Geometry: final body of the model. Coordinates: model frame, mm. A direction names the side the tool comes from. Coordinates: 2 decimals unless noted, no trailing zeros. Write each loop counter-clockwise with the first axis right and the second up, starting at its lowest first coordinate (ties: lowest second). Pieces come first, ordered by that corner, then holes. Notation, with made-up numbers: (4, -1) - (13, -1) arc R16 cw to (13, 8) - close; hole circle Ø4 at (4, 21). An arc over 180 degrees is marked (long way). Put each result on its own line as item: value.
```python
from build123d import *

# Parameters (mm, degrees)
Y_PCB_EXTR_DEPTH                = 1.6
SKETCH1_5_R                     = 1.524
Z0X0_CORNER_EXTR_DEPTH          = 1.6
SKETCH1_6_R                     = 1.524
Z0X_CORNER_EXTR_DEPTH           = 1.6
SKETCH1_7_R                     = 1.524
Z_X0_CORNER_EXTR_DEPTH          = 1.6
SKETCH1_8_R                     = 1.524
Z_X_CORNER_EXTR_DEPTH           = 1.6
Y_DISPLAY_EXTR_DEPTH            = 5.6
SKETCH1_11_W                    = 11.43
SKETCH1_11_H                    = 13.952
Y_DISPLAY_EXTR_BEHIND_USD_DEPTH = 5.6
SKETCH1_12_W                    = 11.43
SKETCH1_12_H                    = 3.048
Y_USD_EXTR_OUTER_EDGE_DEPTH     = 1.6
SKETCH1_13_W                    = 11.43
SKETCH1_13_H                    = 13.952
Y_USD_EXTR_DEPTH                = 2
SKETCH1_14_W                    = 11.43
SKETCH1_14_H                    = 3.048
Y_USD_EXTR_OUTER_BOTTOM_DEPTH   = 2


with BuildPart() as part:
    # Sketch1 → Y_ PCB extr (new body)
    with BuildSketch(Plane(origin=(0, 0, 0), x_dir=(1, 0, 0), z_dir=(0, 1, 0))):
        Polygon((81.28, 50.8), (76.2, 50.8), (66.167, 50.8), (66.167, 47.752), (73.152, 47.752), (73.152, 3.048), (13.716, 3.048), (13.716, 47.752), (54.737, 47.752), (54.737, 50.8), (5.08, 50.8), (0, 50.8), (0, 0), (5.08, 0), (76.2, 0), (81.28, 0), align=None)
    extrude(amount=Y_PCB_EXTR_DEPTH)

    # Sketch1_5 → Z0X0 corner extr (add)
    with BuildSketch(Plane(origin=(0, 0, 0), x_dir=(1, 0, 0), z_dir=(0, 1, 0))):
        with BuildLine():
            Line((0, 50.8), (5.08, 50.8))
            Line((5.08, 50.8), (5.08, 53.98))
            ThreePointArc((5.08, 53.98), (2.54, 56.52), (0, 53.98))
            Line((0, 53.98), (0, 50.8))
        make_face()
        with Locations(Location((2.54, 53.98, 0), (0, 0, 270))):
            Circle(SKETCH1_5_R, mode=Mode.SUBTRACT)
    extrude(amount=Z0X0_CORNER_EXTR_DEPTH)

    # Sketch1_6 → Z0X_ corner extr (add)
    with BuildSketch(Plane(origin=(0, 0, 0), x_dir=(1, 0, 0), z_dir=(0, 1, 0))):
        with BuildLine():
            Line((76.2, 53.98), (76.2, 50.8))
            Line((76.2, 50.8), (81.28, 50.8))
            Line((81.28, 50.8), (81.28, 53.98))
            ThreePointArc((81.28, 53.98), (78.74, 56.52), (76.2, 53.98))
        make_face()
        with Locations(Location((78.74, 53.98, 0), (0, 0, 270))):
            Circle(SKETCH1_6_R, mode=Mode.SUBTRACT)
    extrude(amount=Z0X_CORNER_EXTR_DEPTH)

    # Sketch1_7 → Z_X0 corner extr (add)
    with BuildSketch(Plane(origin=(0, 0, 0), x_dir=(1, 0, 0), z_dir=(0, 1, 0))):
        with BuildLine():
            Line((5.08, -3.18), (5.08, 0))
            Line((5.08, 0), (0, 0))
            Line((0, 0), (0, -3.18))
            ThreePointArc((0, -3.18), (2.54, -5.72), (5.08, -3.18))
        make_face()
        with Locations(Location((2.54, -3.18, 0), (0, 0, 270))):
            Circle(SKETCH1_7_R, mode=Mode.SUBTRACT)
    extrude(amount=Z_X0_CORNER_EXTR_DEPTH)

    # Sketch1_8 → Z_X_ corner extr (add)
    with BuildSketch(Plane(origin=(0, 0, 0), x_dir=(1, 0, 0), z_dir=(0, 1, 0))):
        with BuildLine():
            Line((81.28, -3.18), (81.28, 0))
            Line((81.28, 0), (76.2, 0))
            Line((76.2, 0), (76.2, -3.18))
            ThreePointArc((76.2, -3.18), (78.74, -5.72), (81.28, -3.18))
        make_face()
        with Locations(Location((78.74, -3.18, 0), (0, 0, 270))):
            Circle(SKETCH1_8_R, mode=Mode.SUBTRACT)
    extrude(amount=Z_X_CORNER_EXTR_DEPTH)

    # Sketch1_10 → Y_ display extr (add)
    with BuildSketch(Plane(origin=(0, 0, 0), x_dir=(1, 0, 0), z_dir=(0, 1, 0))):
        Polygon((73.152, 47.752), (66.167, 47.752), (66.167, 33.8), (54.737, 33.8), (54.737, 47.752), (13.716, 47.752), (13.716, 3.048), (73.152, 3.048), align=None)
    extrude(amount=Y_DISPLAY_EXTR_DEPTH)

    # Sketch1_11 → Y_ display extr behind uSD (add)
    with BuildSketch(Plane(origin=(0, 0, 0), x_dir=(1, 0, 0), z_dir=(0, 1, 0))):
        with Locations((60.452, 40.776)):
            Rectangle(SKETCH1_11_W, SKETCH1_11_H)
    extrude(amount=Y_DISPLAY_EXTR_BEHIND_USD_DEPTH)

    # Sketch1_12 → Y- uSD extr outer edge (add)
    with BuildSketch(Plane(origin=(0, 0, 0), x_dir=(1, 0, 0), z_dir=(0, 1, 0))):
        with Locations((60.452, 49.276)):
            Rectangle(SKETCH1_12_W, SKETCH1_12_H)
    extrude(amount=Y_USD_EXTR_OUTER_EDGE_DEPTH)

    # Sketch1_13 → Y- uSD extr (add)
    with BuildSketch(Plane(origin=(0, 0, 0), x_dir=(1, 0, 0), z_dir=(0, 1, 0))):
        with Locations((60.452, 40.776)):
            Rectangle(SKETCH1_13_W, SKETCH1_13_H)
    extrude(amount=-Y_USD_EXTR_DEPTH)

    # Sketch1_14 → Y- uSD extr outer bottom (add)
    with BuildSketch(Plane(origin=(0, 0, 0), x_dir=(1, 0, 0), z_dir=(0, 1, 0))):
        with Locations((60.452, 49.276)):
            Rectangle(SKETCH1_14_W, SKETCH1_14_H)
    extrude(amount=-Y_USD_EXTR_OUTER_BOTTOM_DEPTH)


solid = part.part
```
1. Mould query, pull axis X, two halves, no side actions, for faces 1 (the flat face through (48, 1, -50.8)), 2 (the flat face through (0, 1, -26)), 3 (the flat face through (43, 4, -47.752)), 4 (the flat face through (73.152, 4, -25)). Classes: +X half, -X half, draft (parallel to the pull), parting line (faces both ways), or undercut.
Answer below:
face 1: undercut
face 2: -X half
face 3: draft
face 4: +X half
2. Section query B-B (z = -14). Return loops of the section in (x, y), then the cut area to 3 significant figures.
Answer below:
outline: (0, 0) - (81.28, 0) - (81.28, 1.6) - (73.15, 1.6) - (73.15, 5.6) - (13.72, 5.6) - (13.72, 1.6) - (0, 1.6) - close
area: 368 mm²
3. Section query A-A (x = 78.74). Return loops of the section in (y, z).
Answer below:
outline: (0, -56.52) - (1.6, -56.52) - (1.6, -55.5) - (0, -55.5) - close; (0, -52.46) - (1.6, -52.46) - (1.6, 1.66) - (0, 1.66) - close; (0, 4.7) - (1.6, 4.7) - (1.6, 5.72) - (0, 5.72) - close
4. Section query C-C (x = 58). Return loops of the section in (y, z), then the cut area to 3 significant figures.
Answer below:
outline: (-2, -50.8) - (1.6, -50.8) - (1.6, -47.75) - (5.6, -47.75) - (5.6, -3.05) - (1.6, -3.05) - (1.6, 0) - (0, 0) - (0, -33.8) - (-2, -33.8) - close
area: 294 mm²
5. Section query D-D (y = 4.5). Return loops of the section in (x, z), then the cut area to 3 significant figures.
Answer below:
outline: (13.72, -47.75) - (73.15, -47.75) - (73.15, -3.05) - (13.72, -3.05) - close
area: 2,660 mm²
6. Ray query, probe 1 along Z at (x, y) = (78.74, 0.9); probe 2 along Y at (x, z) = (25.5, -5); probe 3 along Z at (x, y) = (66, 0.75). Return the intervals inside material, ascending. Write a range as from..to.
Answer below:
probe 1: z = -56.52..-55.5, -52.46..1.66, 4.7..5.72
probe 2: y = 0..5.6
probe 3: z = -50.8..0
7. Set-up query: faces 5 (the flat face through (76.2, 1, 2)), 6 (the flat face through (60, -2, -42)), 7 (the cylindrical face through (1.613, 0.789, 1.971)), 8 (the flat face through (60, -1, -33.8)), 9 (the flat face through (76.2, 1, -52)). Return all of +Z, -Z, +X, -X, +Y, -Y with unobstructed straight access to the full face (end or side cutting, diameter ignored); none if empty.
Answer below:
face 5: +Z, +Y, -Y
face 6: +Z, -Z, +X, -X, -Y
face 7: +Y, -Y
face 8: +Z, +X, -X, -Y
face 9: -Z, +Y, -Y
8. Pin query (flat end, axial travel): pin 1 Ø1 at (x, y) = (36.5, 4) entering from +Z; pin 2 Ø3 at (x, y) = (43, -0.5) entering from -Z; pin 3 Ø3.5 at (x, z) = (2.54, 3.18) entering from +Y; pin 4 Ø2.5 at (x, z) = (78.74, -53.98) entering from -Y. Return the tip coordinate at first contact, or that it passes through.
Answer below:
pin 1: stops at z = -3.05
pin 2: stops at z = -50.8
pin 3: stops at y = 1.6
pin 4: passes through
